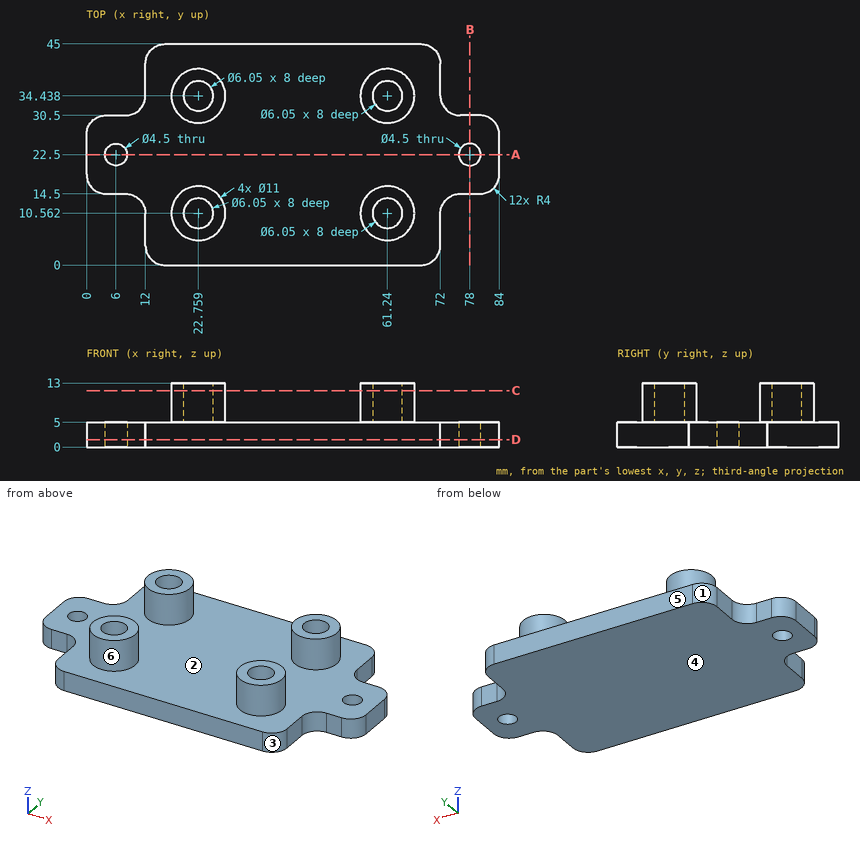
Job drawing, mm, ordinate dimensions from the low corner. One solid piece. A direction names the side the tool comes from. Round coordinates to 2 decimals unless told otherwise and drop trailing zeros. Write each loop counter-clockwise with the first axis right and the second up, starting at its lowest first coordinate (ties: lowest second). Pieces come first, ordered by that corner, then holes.
1) Drill centre lines: probe 1 along Y at (x, z) = (61.5, 8.75) (1 decimal); probe 2 along X at (y, z) = (22, 4) (1 decimal); probe 3 along Y at (x, z) = (25, 6.5) (1 decimal). Where is each one in solid material? Low to high.
2) Band-saw the part on A-A, the plane y = 22.5. List the corners of the cut face in (x, z).
3) Pin check, flat tips, straight feed: pin 1 (3 mm diameter, centred on x = 6.5, z = 2, fed in from -Y); pin 2 (2 mm diameter, centred on y = 32, z = 10.5, fed in from +X); pin 3 (1.5 mm diameter, centred on y = 36.5, z = 3.5, fed in from -X); pin 4 (1.5 mm diameter, centred on y = 23, z = 6.5, fed in from -X). Stop position of each tip, or through.
4) Band-saw the part on D-D, the plane z = 1.5. List the corners of the cut face in (x, y).
5) Band-saw the part on C-C, the plane z = 11.5. Give the number of separate pieces and of enclosed holes in the cut face, and give its area (3 significant figures).
6) Band-saw the part on B-B, the plane x = 78. List the corners of the cut face in (y, z).
7) 3-axis set-ups, long thin cutter, end or side, ignore diameter. For the marked faces 5 and 6: which of +Z, -Z, +X, -X, +Y, -Y reach the whole face in a straight line?
8) Mould opens along X. For the marked faces 1, 2, 3 and 4 say: +X half, -X half, draft (parallel to the pull), parting line (faces both ways), or undercut.
Ans:
1. probe 1: y = 5.1 to 7.5, 13.6 to 16.1, 28.9 to 31.4, 37.5 to 39.9
1. probe 2: x = 0 to 3.8, 8.2 to 75.8, 80.2 to 84
1. probe 3: y = 5.5 to 8.5, 12.6 to 15.6, 29.4 to 32.4, 36.5 to 39.5
2. outline: (0, 0) - (3.75, 0) - (3.75, 5) - (0, 5) - close; (8.25, 0) - (75.75, 0) - (75.75, 5) - (8.25, 5) - close; (80.25, 0) - (84, 0) - (84, 5) - (80.25, 5) - close
3. pin 1: stops at y = 14.5
3. pin 2: stops at x = 66.55
3. pin 3: stops at x = 12
3. pin 4: passes through
4. outline: (0, 18.5) arc R4 ccw to (4, 14.5) - (8, 14.5) arc R4 cw to (12, 10.5) - (12, 4) arc R4 ccw to (16, 0) - (68, 0) arc R4 ccw to (72, 4) - (72, 10.5) arc R4 cw to (76, 14.5) - (80, 14.5) arc R4 ccw to (84, 18.5) - (84, 26.5) arc R4 ccw to (80, 30.5) - (76, 30.5) arc R4 cw to (72, 34.5) - (72, 41) arc R4 ccw to (68, 45) - (16, 45) arc R4 ccw to (12, 41) - (12, 34.5) arc R4 cw to (8, 30.5) - (4, 30.5) arc R4 ccw to (0, 26.5) - close; hole circle Ø4.5 at (6, 22.5); hole circle Ø4.5 at (78, 22.5)
5. separate pieces: 4
5. enclosed holes: 4
5. area: 265 mm2
6. outline: (14.5, 0) - (20.25, 0) - (20.25, 5) - (14.5, 5) - close; (24.75, 0) - (30.5, 0) - (30.5, 5) - (24.75, 5) - close
7. face 5: +Z, -Z, +X, -X, +Y
7. face 6: +Z
8. face 1: -X half
8. face 2: undercut
8. face 3: +X half
8. face 4: draft
